Geometry: final body of the model. Coordinates: model frame, mm. A direction names the side the tool comes from. Coordinates: 2 decimals unless noted, no trailing zeros. Order: outer loops, then holes, each group sorted by start corner. A loop starts at its lowest first (then second) coordinate and runs counter-clockwise, first axis right, second up. Notation, with made-up numbers: M 44.5,-37 L 88.5,-37 A23 cw 88.5,-5 Z; hole C 74,12 d3. An arc over 180 degrees is marked long. One line per question, with ' | ' between items.
from build123d import *

# Parameters (mm, degrees)
SKETCH1_R           = 19.05
BOSS_EXTRUDE1_DEPTH = 1.905
SKETCH6_R           = 5.3
CUT_EXTRUDE2_DEPTH  = 7.35


with BuildPart() as part:
    # Sketch1 → Boss-Extrude1 (new body, symmetric)
    with BuildSketch(Plane(origin=(32.015745885, 0, 0), x_dir=(0, 0, -1), z_dir=(1, 0, 0))):
        with Locations((136.328078847, 49.836172535)):
            Circle(SKETCH1_R)
    extrude(amount=BOSS_EXTRUDE1_DEPTH, both=True)

    # Sketch5 → Revolve1 (revolve)
    with BuildSketch(Plane(origin=(0, 0, -136.328078847), x_dir=(-1, 0, 0), z_dir=(0, 0, -1))):
        Polygon((-32.015745885, 68.886172535), (-33.920745885, 70.791172535), (-35.190745885, 70.791172535), (-35.190745885, 49.836172535), (-33.920745885, 49.836172535), (-33.920745885, 68.886172535), align=None)
    revolve1 = revolve(axis=Axis((33.920745885, 49.836172535, -136.328078847), (-1, 0, 0)))

    # Mirror2: Revolve1 across plane
    add(revolve1.mirror(Plane(origin=(32.015745885, 0, 0), x_dir=(0, 0, 1), z_dir=(1, 0, 0))))

    # Sketch6 → Cut-Extrude2 (cut, through all)
    with BuildSketch(Plane(origin=(35.190745885, 0, 0), x_dir=(0, 0, -1), z_dir=(1, 0, 0))):
        with Locations((136.328078847, 49.836172535)):
            Circle(SKETCH6_R)
    extrude(amount=-CUT_EXTRUDE2_DEPTH, mode=Mode.SUBTRACT)


solid = part.part
1. Draft query along X for faces 1 (the face through (31.9, 47.34, -155.33)), 2 (the face through (28.841, 54, -132)), 3 (the face through (34.56, 59.51, -117.74)). Return one class per face: pulls with the +X half, pulls with the -X half, needs draft (parallel to the pull), parting line crosses it, or undercut.
Response values:
face 1: undercut | face 2: pulls with the -X half | face 3: needs draft
2. Section B-B, the plane x = 34.5. Output: boundary loops of the cut face in (y, z) (3 decimals).
Response values:
outline: C 49.836,-136.328 d41.91; hole C 49.836,-136.328 d10.6
3. Section A-A, the plane x = 31.25. Output: boundary loops of the cut face in (y, z), and give its area (3 significant figures).
Response values:
outline: C 49.84,-136.33 d39.63; hole C 49.84,-136.33 d10.6 | area: 1,150 mm^2
4. Material intervals for line 1 (Z direction, x = 30, y = 52.5); line 2 (Z direction, x = 33.25, y = 51.5); line 3 (Y direction, x = 29.75, z = -135.5), sorted ascending. Write a range as [from, to].
Response values:
line 1: z = [-157.11, -140.91], [-131.75, -115.54] | line 2: z = [-156.54, -141.36], [-131.3, -116.11] | line 3: y = [28.9, 44.6], [55.07, 70.77]
5. Pin query (flat end, axial travel): P1, Ø2, axis at x = 34, z = -146.5, coming from the -Y side; P2, Ø1.5, axis at x = 33.5, y = 60, coming from the -Z side; P3, Ø1, axis at x = 30, y = 34, coming from the -Z side. Return the tip coordinate at first contact, or that it passes through.
Response values:
P1: stops at y = 31 | P2: stops at z = -154.98 | P3: stops at z = -150.61
6. Access query for faces 4 (the face through (32.06, 51.428, -141.383)), 5 (the face through (32.13, 47.34, -155.33)). Directions: +Z, -Z, +X, -X, +Y, -Y. A direction counts if a zero-diameter tool reaches every point of the face in a straight line with its end or side. Return the directions, or none.
Response values:
face 4: +X, -X | face 5: none
